Job drawing, mm, ordinate dimensions from the low corner. One solid piece. A direction names the side the tool comes from. Coordinates: 2 decimals unless noted, no trailing zeros. Loops run counter-clockwise (first coordinate to the right, second up) from the corner with the lowest first, then second, coordinate; pieces in that order, holes last. Notation, with made-up numbers: (82, 22.25) - (100, 22.25) arc R8 ccw to (100, 30.25) - close; hole circle Ø10 at (-8, -23). An arc over 180 degrees is marked (long way). One line per question, with ' | ' between items. Start each with the question number.
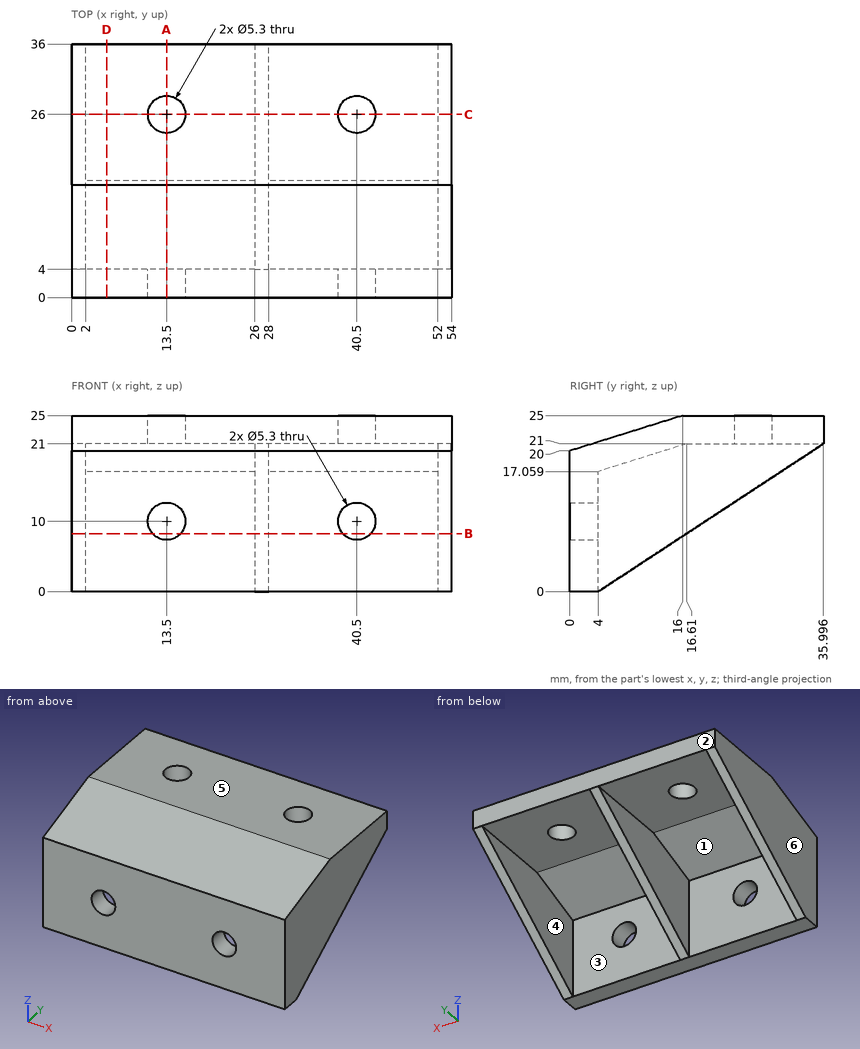
1) Band-saw the part on B-B on z = 8.25. List the corners of the cut face in (x, y).
2) Wall check: line 1 along X through (y, z) = (16, 12.5); line 2 along Y through (x, z) = (51, 10.5); line 3 along Z through (x, y) = (20, 31). Give the ranges that are in metal, low to high. Write a range as [from, to].
3) Mould opens along X. For the marked faces 3, 4, 5 and 6 say: +X half, -X half, draft (parallel to the pull), parting line (faces both ways), or undercut.
4) Tool access for the marked faces 1 and 2: list every direction of +Z, -Z, +X, -X, +Y, -Y with a clear straight run to the whole face (end or side of a thin tool).
5) Band-saw the part on A-A on x = 13.5. List the corners of the cut face in (y, z).
6) Pin check, flat tips, straight feed: pin 1 Ø6 at (x, y) = (28, 26.5) entering from -Z; pin 2 Ø5 at (x, z) = (13.5, 10) entering from -Y; pin 3 Ø8.5 at (x, z) = (19, 5) entering from +Y; pin 4 Ø6 at (x, y) = (12, 32) entering from -Z. Stop position of each tip, or through.
7) Band-saw the part on D-D on x = 5. List the corners of the cut face in (y, z), then the cut area to 3 significant figures.
8) Band-saw the part on C-C on y = 26. List the corners of the cut face in (x, z).
Values found:
1) outline: (0, 0) - (11.51, 0) - (11.51, 4) - (2, 4) - (2, 16.57) - (0, 16.57) - close; (15.49, 0) - (38.51, 0) - (38.51, 4) - (28, 4) - (28, 16.57) - (26, 16.57) - (26, 4) - (15.49, 4) - close; (42.49, 0) - (54, 0) - (54, 16.57) - (52, 16.57) - (52, 4) - (42.49, 4) - close
2) line 1: [0, 2], [26, 28], [52, 54] | line 2: [0, 4] | line 3: [21, 25]
3) face 3: undercut | face 4: undercut | face 5: draft | face 6: -X half
4) face 1: -Z, +Y | face 2: +Z, -Z, +X, -X, +Y
5) outline: (0, 0) - (4, 0) - (4, 7.35) - (0, 7.35) - close; (0, 12.65) - (4, 12.65) - (4, 17.06) - (16.61, 21) - (23.35, 21) - (23.35, 25) - (16, 25) - (0, 20) - close; (28.65, 21) - (36, 21) - (36, 25) - (28.65, 25) - close
6) pin 1: z = 12.8 | pin 2: through | pin 3: y = 4 | pin 4: z = 21
7) outline: (0, 0) - (4, 0) - (4, 17.06) - (16.61, 21) - (36, 21) - (36, 25) - (16, 25) - (0, 20) - close | area: 213 mm²
8) outline: (0, 14.44) - (2, 14.44) - (2, 21) - (10.85, 21) - (10.85, 25) - (0, 25) - close; (16.15, 21) - (26, 21) - (26, 14.44) - (28, 14.44) - (28, 21) - (37.85, 21) - (37.85, 25) - (16.15, 25) - close; (43.15, 21) - (52, 21) - (52, 14.44) - (54, 14.44) - (54, 25) - (43.15, 25) - close
